Geometry: final body of the model. Coordinates: model frame, mm. A direction names the side the tool comes from. Coordinates: 2 decimals unless noted, no trailing zeros. Write each loop counter-clockwise with the first axis right and the second up, starting at its lowest first coordinate (ties: lowest second). Pieces come first, ordered by that corner, then holes. Notation, with made-up numbers: M -24.75,89.5 L -6.75,89.5 A30 ccw -6.75,112.5 Z; hole C -17.75,19 d9. An arc over 180 degrees is marked long. Write item = value, one per line. Start each with the question number.
Item 1: Ray query, L1, parallel to Y at x = 407, z = 0.4; L2, parallel to Y at x = 402, z = 4; L3, parallel to Y at x = 405.5, z = 1.7. Return the intervals inside material, ascending. Write a range as [from, to].
Item 2: First-contact query: pin 1 Ø3 at (y, z) = (556, 3) entering from +X; pin 2 Ø1 at (x, z) = (412.5, 2.5) entering from +Y; pin 3 Ø1 at (y, z) = (539.5, 4.5) entering from -X; pin 4 Ø1.7 at (x, y) = (425.56, 544.64) entering from -Z (3 decimals). Flat tips, straight axial feed; report the tip coordinate or a pass-through.
Item 3: Section D-D on y = 558. Output: boundary loops of the cut face in (x, z), plus the area to 3 significant figures.
Item 4: Pull-direction query (X, two-part tool) for faces 1 (the flat face through (387.555, 544, 3)), 2 (the cylindrical face through (428.674, 544.707, 2.884)), 3 (the flat face through (400, 526.389, 3)), 4 (the flat face through (405, 548.139, 3)); classes: +X half, -X half, draft (parallel to the pull), parting line (faces both ways), or undercut.
Item 5: Section B-B on x = 404. Output: boundary loops of the cut face in (y, z).
Item 6: Section C-C on y = 542. Output: boundary loops of the cut face in (x, z).
Item 7: Reachability of faces 5 (the flat face through (403.8, 540.8, 0)), 6 (the flat face through (410, 532, 1)), 7 (the flat face through (405, 535.489, 3)) from +Z, -Z, +X, -X, +Y, -Y: full face, straight path, thin tool, end or side. Return the list, or none.
Item 8: Section A-A on x = 397. Output: boundary loops of the cut face in (y, z), plus the area to 3 significant figures.
from build123d import *

# Parameters (mm, degrees)
SKETCH1_R           = 1.45
SKETCH1_W           = 3.400011
SKETCH1_H           = 6.1
BOSS_EXTRUDE2_DEPTH = 5.85
SKETCH2_R           = 1.25
CUT_EXTRUDE1_DEPTH  = 1


with BuildPart() as part:
    # Sketch1 → Boss-Extrude2 (new body)
    with BuildSketch(Plane.XY):
        with BuildLine():
            Line((388.984643017, 562.888903138), (410.424633118, 562.888903138))
            ThreePointArc((410.424633118, 562.888903138), (412.211329852, 562.148829119), (412.95140387, 560.362132386))
            ThreePointArc((412.95140387, 560.362132386), (416.644097047, 551.447182437), (425.559046996, 547.75448926))
            ThreePointArc((425.559046996, 547.75448926), (428.674633119, 544.638903138), (425.559046996, 541.523317015))
            ThreePointArc((425.559046996, 541.523317015), (416.644097047, 537.830623838), (412.95140387, 528.915673889))
            ThreePointArc((412.95140387, 528.915673889), (412.211329852, 527.128977156), (410.424633118, 526.388903138))
            Line((410.424633118, 526.388903138), (388.984643017, 526.388903138))
            add(Edge.make_bspline(
                [(387.555122745, 527.816961526), (387.476445389, 526.388903138), (388.984643017, 526.388903138)],
                knots=[0, 0, 0, 1, 1, 1], degree=2))
            Line((387.555122745, 527.816961526), (387.555122745, 561.460844041))
            add(Edge.make_bspline(
                [(387.555122745, 561.460844041), (387.476444597, 562.888903138), (388.984643017, 562.888903138)],
                knots=[0, 0, 0, 1, 1, 1], degree=2))
        make_face()
        with Locations((425.559046996, 544.638903138)):
            Circle(SKETCH1_R, mode=Mode.SUBTRACT)
        with Locations((399.559046996, 532.438903138)):
            Circle(SKETCH1_R, mode=Mode.SUBTRACT)
        Polygon((405.566920996, 551.188903138), (405.566920996, 553.788903138), (408.562971247, 553.788903138), (408.562971247, 559.888903138), (402.762971247, 559.888903138), (402.762971247, 553.788903138), (396.355122745, 553.788903138), (396.355122745, 559.888903138), (390.555122745, 559.888903138), (390.555122745, 553.788903138), (393.551172996, 553.788903138), (393.551172996, 551.188903138), align=None, mode=Mode.SUBTRACT)
        with Locations((394.409041496, 532.438903138)):
            Rectangle(SKETCH1_W, SKETCH1_H, mode=Mode.SUBTRACT)
        with Locations((404.709052496, 532.438903138)):
            Rectangle(SKETCH1_W, SKETCH1_H, mode=Mode.SUBTRACT)
        with BuildLine():
            Line((396.165690223, 548.138903138), (413.915690223, 548.138903138))
            ThreePointArc((413.915690223, 548.138903138), (417.415690223, 544.638903138), (413.915690223, 541.138903138))
            Line((413.915690223, 541.138903138), (396.165690223, 541.138903138))
            ThreePointArc((396.165690223, 541.138903138), (392.665690223, 544.638903138), (396.165690223, 548.138903138))
        make_face(mode=Mode.SUBTRACT)
    extrude(amount=BOSS_EXTRUDE2_DEPTH)

    # Sketch2 → Cut-Extrude1 (cut)
    with BuildSketch(Plane.XY):
        with Locations((409.659057996, 532.438903138)):
            Circle(SKETCH2_R)
    extrude(amount=CUT_EXTRUDE1_DEPTH, mode=Mode.SUBTRACT)


solid = part.part
Responses:
q1.L1 = [526.39, 541.14], [548.14, 553.79], [559.89, 562.89]
q1.L2 = [526.39, 541.14], [548.14, 551.19], [553.79, 562.89]
q1.L3 = [526.39, 529.39], [535.49, 541.14], [548.14, 551.19], [559.89, 562.89]
q2.pin_1 = 414.4
q2.pin_2 = 562.34
q2.pin_3 = 387.56
q2.pin_4 = through
q3.outline = M 387.56,0 L 390.56,0 L 390.56,5.85 L 387.56,5.85 Z; M 396.36,0 L 402.76,0 L 402.76,5.85 L 396.36,5.85 Z; M 408.56,0 L 413.17,0 L 413.17,5.85 L 408.56,5.85 Z
q3.area = 82.0 mm²
q4.face_1 = -X half
q4.face_2 = +X half
q4.face_3 = draft
q4.face_4 = undercut
q5.outline = M 526.39,0 L 529.39,0 L 529.39,5.85 L 526.39,5.85 Z; M 535.49,0 L 541.14,0 L 541.14,5.85 L 535.49,5.85 Z; M 548.14,0 L 551.19,0 L 551.19,5.85 L 548.14,5.85 Z; M 559.89,0 L 562.89,0 L 562.89,5.85 L 559.89,5.85 Z
q6.outline = M 387.56,0 L 393.87,0 L 393.87,5.85 L 387.56,5.85 Z; M 416.21,0 L 427.22,0 L 427.22,5.85 L 416.21,5.85 Z
q7.face_5 = -Z, +X, -X, +Y, -Y
q7.face_6 = -Z
q7.face_7 = +Z, -Z
q8.outline = M 526.39,0 L 541.14,0 L 541.14,5.85 L 526.39,5.85 Z; M 548.14,0 L 551.19,0 L 551.19,5.85 L 548.14,5.85 Z; M 553.79,0 L 562.89,0 L 562.89,5.85 L 553.79,5.85 Z
q8.area = 157 mm²
